Autodesk Inventor part; units mm, degrees
ref_plane "YZ Plane" through (0, 0, 0) normal (1, 0, 0) x (0, 1, 0)
ref_plane "XZ Plane" through (0, 0, 0) normal (0, 1, 0) x (-1, 0, 0)
ref_plane "XY Plane" through (0, 0, 0) normal (0, 0, 1) x (1, 0, 0)
sketch "Sketch1" plane through (0, 0, 0) normal (0, 0, 1) x (1, 0, 0)
  line L0 (0, 0) -> (152.4, 0)
  line L1 (152.4, 0) -> (152.4, 76.2)
  line L2 (152.4, 76.2) -> (0, 76.2)
  line L3 (0, 76.2) -> (0, 0)
  dimension "d0" = 152.4
  dimension "d1" = 76.2
extrude "Extrusion1" add sketch "Sketch1" along normal blind 1174.2928
shell "Shell1" thickness 6.35 removed faces 2 at (50.8, 50.8, 0) at (50.8, 50.8, 1174.2928)
sketch "Sketch2" plane through (0, 76.2, 0) normal (0, 1, 0) x (1, 0, 0)
  circle A0 centre (124.9, -1067.1428) radius 3
  circle A1 centre (124.9, -1007.1428) radius 3
  circle A2 centre (124.9, -947.1428) radius 3
  circle A3 centre (124.9, -887.1428) radius 3
  circle A4 centre (124.9, -827.1428) radius 3
  circle A5 centre (124.9, -767.1428) radius 3
  circle A6 centre (124.9, -707.1428) radius 3
  circle A7 centre (124.9, -647.1428) radius 3
  circle A8 centre (124.9, -587.1428) radius 3
  circle A9 centre (124.9, -527.1428) radius 3
  circle A10 centre (124.9, -467.1428) radius 3
  circle A11 centre (124.9, -407.1428) radius 3
  circle A12 centre (124.9, -347.1428) radius 3
  circle A13 centre (124.9, -287.1428) radius 3
  circle A14 centre (124.9, -227.1428) radius 3
  circle A15 centre (124.9, -167.1428) radius 3
  circle A16 centre (124.9, -107.1428) radius 3
  line L0 (114.9, -87.1428) -> (134.9, -87.1428)
  line L1 (134.9, -87.1428) -> (134.9, -1087.1428)
  line L2 (114.9, -1087.1428) -> (134.9, -1087.1428)
  line L3 (114.9, -87.1428) -> (114.9, -1087.1428)
  circle A17 centre (19.9, -1067.1428) radius 3
  circle A18 centre (19.9, -1007.1428) radius 3
  circle A19 centre (19.9, -947.1428) radius 3
  circle A20 centre (19.9, -887.1428) radius 3
  circle A21 centre (19.9, -827.1428) radius 3
  circle A22 centre (19.9, -767.1428) radius 3
  circle A23 centre (19.9, -707.1428) radius 3
  circle A24 centre (19.9, -647.1428) radius 3
  circle A25 centre (19.9, -587.1428) radius 3
  circle A26 centre (19.9, -527.1428) radius 3
  circle A27 centre (19.9, -467.1428) radius 3
  circle A28 centre (19.9, -407.1428) radius 3
  circle A29 centre (19.9, -347.1428) radius 3
  circle A30 centre (19.9, -287.1428) radius 3
  circle A31 centre (19.9, -227.1428) radius 3
  circle A32 centre (19.9, -167.1428) radius 3
  circle A33 centre (19.9, -107.1428) radius 3
  line L4 (9.9, -87.1428) -> (29.9, -87.1428)
  line L5 (29.9, -87.1428) -> (29.9, -1087.1428)
  line L6 (9.9, -1087.1428) -> (29.9, -1087.1428)
  line L7 (9.9, -87.1428) -> (9.9, -1087.1428)
  point P0 (0, 0)
extrude "Extrusion2" cut sketch "Sketch2" against normal up to surface (6.35 mm away) contours A0 | A1 | A2 | A3 | A4 | A5 | A6 | A7 | A8 | A9 | A10 | A11 | A12 | A13 | A14 | A15 | A16 | A17 | A18 | A19 | A20 | A21 | A22 | A23 | A24 | A25 | A26 | A27 | A28 | A29 | A30 | A31 | A32 | A33
properties part number "HORIZONTALTUBE"
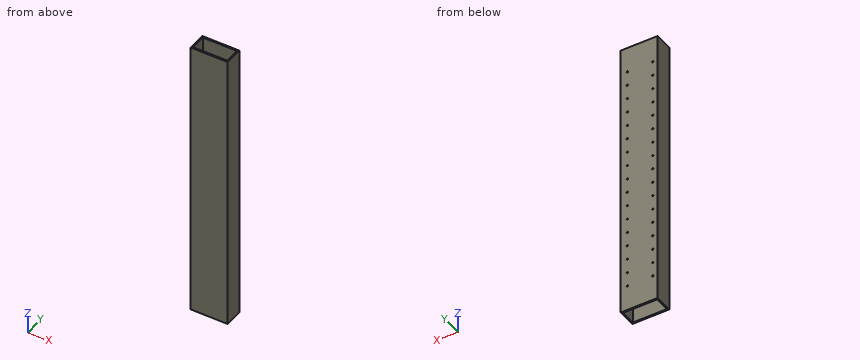
Input: part model. Units: mm. Frame: model coordinates. Coordinates: 2 decimals unless noted, no trailing zeros. Write each loop counter-clockwise with the first axis right and the second up, starting at its lowest first coordinate (ties: lowest second). Pieces come first, ordered by that corner, then holes. Notation, with made-up numbers: (-3.75, 11) - (52.25, 11) arc R19 ccw to (52.25, 42) - close; hole circle Ø9 at (-35, 43.5). An arc over 180 degrees is marked (long way). Put each result on its own line as item: value. Start each with the question number.
1) Ray query, L1, parallel to Y at x = 134, z = 743; L2, parallel to X at y = 43, z = 959.5. Return the intervals inside material, ascending.
2) Cut plane A-A (y = 21.5). Return the cut outline in (x, z), plus the area to 3 significant figures.
3) Contact query for flat-ended pins moving along their axis: pin 1 (5.5 mm diameter, centred on x = 124.9, z = 347.14, fed in from +Y); pin 2 (4 mm diameter, centred on x = 48.5, y = 9.5, fed in from +Z). Output: stop coordinate, or through.
4) Cut plane B-B (x = 39). Return the cut outline in (y, z), plus the area to 3 significant figures.
5) Cut plane C-C (z = 503). Return the cut outline in (x, y).
Resolved:
1. L1: y = 0 to 6.35, 69.85 to 76.2
1. L2: x = 0 to 6.35, 146.05 to 152.4
2. outline: (0, 0) - (6.35, 0) - (6.35, 1174.29) - (0, 1174.29) - close; (146.05, 0) - (152.4, 0) - (152.4, 1174.29) - (146.05, 1174.29) - close
2. area: 14,900 mm2
3. pin 1: stops at y = 6.35
3. pin 2: passes through
4. outline: (0, 0) - (6.35, 0) - (6.35, 1174.29) - (0, 1174.29) - close; (69.85, 0) - (76.2, 0) - (76.2, 1174.29) - (69.85, 1174.29) - close
4. area: 14,900 mm2
5. outline: (0, 0) - (152.4, 0) - (152.4, 76.2) - (0, 76.2) - close; hole (6.35, 6.35) - (146.05, 6.35) - (146.05, 69.85) - (6.35, 69.85) - close
